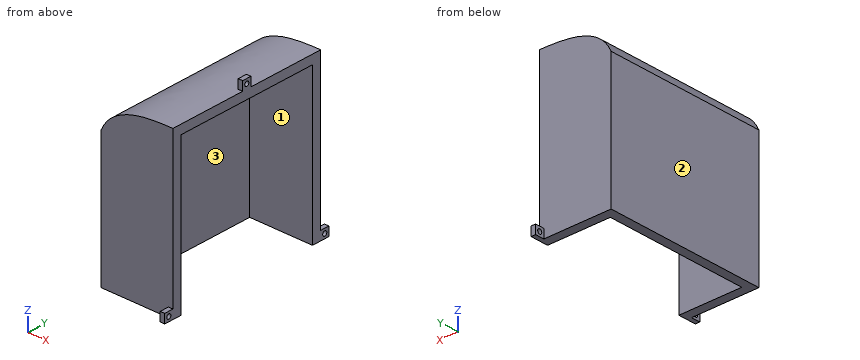
from build123d import *

# Parameters (mm, degrees)
F1_DEPTH = 114.3
F2_T     = -6.35
F3_W     = 6.35
F3_H     = 6.35
F3_R     = 1.5875
F4_DEPTH = 3.175


with BuildPart() as f1:
    # F0 (on Front) → F1 (new body)
    with BuildSketch(Plane.XZ):
        with BuildLine():
            Line((0, -31.3225934026), (0, 82.9774065974))
            add(Edge.make_bspline(
                [(-50.8, 62.9390975716), (-47.0688648848, 71.4759068336), (-33.0013413264, 81.0637344093), (-15.4475548971, 82.9055417219), (0, 82.9774065974)],
                knots=[0, 0, 0, 0, 0.4529279664, 1, 1, 1, 1], degree=3))
            Line((-50.8, 62.9390975716), (-50.8, -31.3225934026))
            Line((-50.8, -31.3225934026), (0, -31.3225934026))
        make_face()
    extrude(amount=F1_DEPTH)

    # F2
    f2_openings = [f1.faces().sort_by_distance(p)[0] for p in [
        (0, -57.15, 25.827407),
        (-25.4, -57.15, -31.322593),
    ]]
    offset(amount=F2_T, openings=f2_openings, kind=Kind.INTERSECTION)

    # F3 (on Right) → F4 (join)
    with BuildSketch(Plane.YZ):
        with Locations((3.175, -28.1475934026)):
            Rectangle(F3_W, F3_H)
        with Locations((3.175, -28.1475934026)):
            Circle(F3_R, mode=Mode.SUBTRACT)
        with Locations((-117.475, -28.1475934026)):
            Rectangle(F3_W, F3_H)
        with Locations((-117.475, -28.1475934026)):
            Circle(F3_R, mode=Mode.SUBTRACT)
        Polygon((-53.975, 89.3274065974), (-60.325, 89.3274065974), (-60.325, 82.9774065974), (-60.325, 81.7074065974), (-53.975, 81.7074065974), (-53.975, 82.9774065974), align=None)
        with Locations((-57.15, 86.1524065974)):
            Circle(F3_R, mode=Mode.SUBTRACT)
    extrude(amount=-F4_DEPTH)


solid = f1.part
Here's how the part is built. I have some questions about the finished solid (model axes, mm). Face numbers are marked on the shaded views. Round coordinates to 2 decimals unless told otherwise and drop trailing zeros. Order: outer loops, then holes, each group sorted by start corner. A loop starts at its lowest first (then second) coordinate and runs counter-clockwise, first axis right, second up. Notation, with made-up numbers: M 0,73 L 26,73 A8 ccw 26,77 Z; hole C -33,41 d3. An arc over 180 degrees is marked long. Return JSON: item names as keys, results as strings. Group by question number.
1. If we section it at A-A on z = -14: List the corners of the cut face in (x, y) for me.
2. If we mould it in two halves opening along Y, with no side actions, what happens to the marked faces 1, 2 and 3? For each: pulls with the +Y half, pulls with the -Y half, needs draft (parallel to the pull), parting line crosses it, or undercut.
3. I'm going to push flat-ended pins straight in: pin 1 Ø1.5 at (x, y) = (-6.5, -49) entering from -Z; pin 2 Ø2.5 at (x, y) = (-1.5, 4.5) entering from +Z; pin 3 Ø8 at (x, y) = (-20.5, -44) entering from -Z. Where does each tip first touch, or does it pass through?
4. Please list where these lines run through material, in increasing order: probe 1 along Y at (x, z) = (-18, 56); probe 2 along Z at (x, y) = (-1.7, -57.15).
Reply:
{
 "1": {"outline": "M -50.8,-114.3 L 0,-114.3 L 0,-107.95 L -44.45,-107.95 L -44.45,-6.35 L 0,-6.35 L 0,0 L -50.8,0 Z"},
 "2": {"face 1": "undercut", "face 2": "needs draft", "face 3": "undercut"},
 "3": {"pin 1": "z = 76.5", "pin 2": "z = -24.97", "pin 3": "z = 74.69"},
 "4": {"probe 1": "-114.3 to -107.95, -6.35 to 0", "probe 2": "76.62 to 84.56, 87.74 to 89.33"}
}
